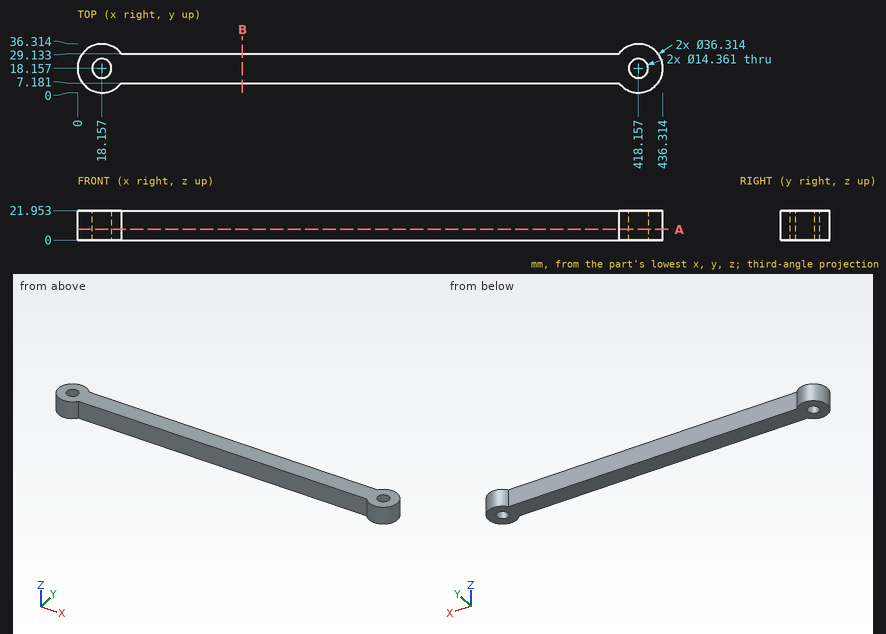
Input: dimensioned drawing with shaded views. Units: mm. Origin: part minimum x, y, z. Coordinates: 2 decimals unless noted, no trailing zeros. Write each loop counter-clockwise with the first axis right and the second up, starting at its lowest first coordinate (ties: lowest second). Pieces come first, ordered by that corner, then holes. Notation, with made-up numbers: (78.25, 28.5) -> (122.25, 28.5) arc R14 cw to (122.25, 51.5) -> close; hole circle Ø9 at (-36, -6.5). An arc over 180 degrees is marked (long way). Return JSON: item names as keys, results as strings. Group by question number.
1) Section query B-B, the plane x = 123. Return loops of the section in (y, z).
2) Ray query, line 1 along X through (y, z) = (18, 13) (1 decimal); line 2 along X through (y, z) = (20, 10.25) (1 decimal); line 3 along Y through (x, z) = (338.5, 10.75). Return the intervals inside material, ascending.
3) Contact query for flat-ended pins moving along their axis: P1, Ø8, axis at y = 6.5, z = 14, coming from the -X side; P2, Ø3, axis at x = 293, z = 4.5, coming from the +Y side; P3, Ø4, axis at y = 32, z = 2, coming from the -X side (1 decimal). Output: stop coordinate, or through.
4) Section query A-A, the plane z = 8. Return loops of the section in (x, y).
From the geometry:
{
 "1": {"outline": "(7.18, 0) -> (29.13, 0) -> (29.13, 21.95) -> (7.18, 21.95) -> close"},
 "2": {"line 1": "0 to 11, 25.3 to 411, 425.3 to 436.3", "line 2": "0.1 to 11.2, 25.1 to 411.2, 425.1 to 436.2", "line 3": "7.18 to 29.13"},
 "3": {"P1": "x = 1.69", "P2": "y = 29.13", "P3": "x = 4.4"},
 "4": {"outline": "(32.62, 7.18) -> (403.69, 7.18) arc R18.16 ccw (long way) to (403.69, 29.13) -> (32.62, 29.13) arc R18.16 ccw (long way) to start; hole circle Ø14.36 at (18.16, 18.16); hole circle Ø14.36 at (418.16, 18.16)"}
}
